Source: CAD feature listing. Evaluate the final solid. Frame: model axes, mm. A direction names the side the tool comes from. Give positions to 0.01 mm unless a question says otherwise; leave off trailing zeros. Loops run counter-clockwise (first coordinate to the right, second up) from the corner with the lowest first, then second, coordinate; pieces in that order, holes last. Notation, with made-up numbers: M -20.5,-10.75 L 28.5,-10.75 A32 cw 28.5,25.25 Z; hole C -4.75,39 d6. An arc over 180 degrees is marked long. Put each result on its own line as item: value.
Autodesk Inventor part; units mm, degrees
ref_plane "YZ Plane" through (0, 0, 0) normal (1, 0, 0) x (0, 1, 0)
ref_plane "XZ Plane" through (0, 0, 0) normal (0, 1, 0) x (-1, 0, 0)
ref_plane "XY Plane" through (0, 0, 0) normal (0, 0, 1) x (1, 0, 0)
sketch "Sketch1" plane through (0, 0, 0) normal (0, 0, 1) x (1, 0, 0)
  line L0 (0, 0) -> (80, 0)
  circle A0 centre (40, 15) radius 3.5
  line L1 (0, 0) -> (0, 30)
  line L2 (0, 30) -> (80, 30)
  line L3 (80, 30) -> (80, 0)
  point P0 (40, 0)
  dimension "d0" = 80
  dimension "d2" = 7
  dimension "d3" = 15
  dimension "d4" = 30
extrude "Extrusion1" add sketch "Sketch1" along normal blind 5
sketch "Sketch2" plane through (0, 0, 5) normal (0, 0, 1) x (1, 0, 0)
  line L0 (0, 0) -> (80, 0)
  line L1 (0, 0) -> (80, 0)
  line L2 (80, 0) -> (80, 5)
  line L3 (80, 5) -> (0, 5)
  line L4 (0, 5) -> (0, 0)
  line L5 (80, 0) -> (80, 30)
  point P0 (40, 0)
  dimension "d8" = 5
extrude "Extrusion2" add sketch "Sketch2" along normal blind 15
sketch "Sketch3" plane through (0, 0, 5) normal (0, 0, 1) x (1, 0, 0)
  circle A0 centre (31.5, 15) radius 2
  circle A1 centre (48.5, 15) radius 2
  line L0 (80, 5) -> (80, 30)
  line L1 (80, 30) -> (0, 30)
  line L2 (0, 30) -> (0, 5)
  line L3 (0, 5) -> (80, 5)
  circle A2 centre (40, 15) radius 3.5
  line L4 (31.5, 15) -> (48.5, 15) construction
  point P0 (0, 0)
  dimension "d11" = 4
  dimension "d12" = 4
  dimension "d13" = 17
extrude "Extrusion3" cut sketch "Sketch3" against normal through all contours A0 | A1
sketch "Sketch5" plane through (0, 5, 5) normal (0, 1, 0) x (1, 0, 0)
  line L0 (0, 0) -> (0, -15) construction
  line L1 (80, 5) -> (80, -15) construction
  circle A0 centre (20, -7.5) radius 3
  circle A1 centre (40, -7.5) radius 3
  circle A2 centre (60, -7.5) radius 3
  line L2 (0, -7.5) -> (80, -7.5) construction
  point P0 (0, 5)
  point P1 (40, -7.5)
  point P2 (40, -7.5)
  dimension "d17" = 6
  dimension "d18" = 6
  dimension "d19" = 20
  dimension "d25" = 6
  dimension "d26" = 20
extrude "Extrusion4" cut sketch "Sketch5" against normal through all
sketch "Sketch6" plane through (0, 0, 5) normal (0, 0, 1) x (1, 0, 0)
  circle A0 centre (40, 15) radius 3.5
  circle A1 centre (40, 15) radius 12.5
  point P0 (0, 0)
  dimension "d27" = 25
extrude "Extrusion5" cut sketch "Sketch6" along normal through all
sketch "Sketch8" plane through (80, 0, 0) normal (1, 0, 0) x (0, 0, -1)
  line L0 (-5, 5) -> (-20, 5)
  line L1 (-5, 5) -> (-5, 30)
  line L2 (-20, 5) -> (-5, 30)
  line L3 (-5, 30) -> (-5, 5)
  line L4 (-5, 5) -> (-20, 5)
  point P0 (0, 0)
extrude "Extrusion6" add sketch "Sketch8" against normal blind 10
sketch "Sketch9" plane through (0, 0, 0) normal (-1, 0, 0) x (0, 0, 1)
  line L0 (20, 0) -> (20, 5)
  line L1 (20, 5) -> (5, 30)
  line L2 (5, 5) -> (20, 5)
  line L3 (5, 30) -> (5, 5)
  line L4 (5, 5) -> (20, 5)
  point P0 (0, 0)
extrude "Extrusion7" add sketch "Sketch9" against normal blind 10
properties part number "C005" material "ABS Plastic"
1. Section query C-C (z = 11.25). Output: boundary loops of the cut face in (x, y), plus the area to 3 significant figures.
Found:
outline: M 0,0 L 17.27,0 L 17.27,5 L 10,5 L 10,19.58 L 0,19.58 Z; M 22.73,0 L 37.27,0 L 37.27,2.8 A12.5 cw 32.5,5 L 22.73,5 Z; M 42.73,0 L 57.27,0 L 57.27,5 L 47.5,5 A12.5 cw 42.73,2.8 Z; M 62.73,0 L 80,0 L 80,19.58 L 70,19.58 L 70,5 L 62.73,5 Z
area: 597 mm^2
2. Section query D-D (x = 40). Output: boundary loops of the cut face in (y, z), plus the area to 4 significant figures.
Found:
outline: M 0,0 L 11.5,0 L 11.5,5 L 2.5,5 L 2.5,9.5 L 0,9.5 Z; M 0,15.5 L 2.5,15.5 L 2.5,20 L 0,20 Z; M 18.5,0 L 30,0 L 30,5 L 18.5,5 Z
area: 137.5 mm^2
3. Contact query for a flat-ended pin moving along its axis: P1, Ø7.5, axis at x = 22, z = 11.5, coming from the +Y side. Output: stop coordinate, or through.
Found:
P1: y = 5
4. Section query A-A (y = 15). Output: boundary loops of the cut face in (x, z).
Found:
outline: M 0,0 L 29.5,0 L 29.5,5 L 10,5 L 10,14 L 0,14 Z; M 33.5,0 L 36.5,0 L 36.5,5 L 33.5,5 Z; M 43.5,0 L 46.5,0 L 46.5,5 L 43.5,5 Z; M 50.5,0 L 80,0 L 80,14 L 70,14 L 70,5 L 50.5,5 Z
5. Draft query along Z for faces 1 (the flat face through (24, 5, 12)), 2 (the flat face through (39, 2, 20)), 3 (the cylindrical face through (57, 2.5, 12.4)). Return one class per face: pulls with the +Z half, pulls with the -Z half, needs draft (parallel to the pull), parting line crosses it, or undercut.
Found:
face 1: needs draft
face 2: pulls with the +Z half
face 3: undercut
6. Material intervals for line 1 (X direction, y = 2.1, z = 12.5); line 2 (Y direction, x = 31.5, z = 1.65); line 3 (Z direction, x = 60, y = 3.2), sorted ascending. Write a range as from..to.
Found:
line 1: 0..17, 23..37, 43..57, 63..80
line 2: 0..13, 17..30
line 3: 0..9.5, 15.5..20
7. Section query B-B (x = 48.5). Output: boundary loops of the cut face in (y, z).
Found:
outline: M 0,0 L 13,0 L 13,5 L 5,5 L 5,20 L 0,20 Z; M 17,0 L 30,0 L 30,5 L 17,5 Z
8. Access query for faces 4 (the cylindrical face through (33.408, 15.601, 2.535)), 5 (the flat face through (40, 19, 5)). Directions: +Z, -Z, +X, -X, +Y, -Y. A direction counts if a zero-diameter tool reaches every point of the face in a straight line with its end or side. Return the directions, or none.
Found:
face 4: +Z, -Z
face 5: +Z, +Y
